Read the model definition and answer for the solid it produces. Units are mm, in the model's axes. A direction names the side the tool comes from. Give positions to 0.01 mm unless a question says otherwise; leave off trailing zeros. Write each loop counter-clockwise with the first axis right and the second up, starting at its lowest first coordinate (ties: lowest second). Pieces come first, ordered by that corner, then holes. Notation, with made-up numbers: M 9.25,49 L 58.25,49 A20 ccw 58.25,63 Z; hole C 49.5,-13.75 d7. An arc over 180 degrees is marked long. Write each question's results on one line, items separated by ' | '. Start each with the question number.
```python
from build123d import *
from build123d.topology import SkipClean

# Parameters (mm, degrees)
SKETCH_1_W               = 49.5
SKETCH_1_H               = 24.5
EXTRUDE_1_DEPTH          = 36
SKETCH_2_R               = 2.5
CUT_EXTRUDE_1_DEPTH      = 3
SKETCH_3_W               = 15.2
SKETCH_3_H               = 2.5
CUT_EXTRUDE_2_DEPTH      = 12
FILLET_1_R               = 3
CUT_EXTRUDE_3_DEPTH      = 46.372072908
CUT_EXTRUDE_3_DEPTH_BACK = 46.372072908
SKETCH_5_R               = 1.95
CUT_EXTRUDE_4_DEPTH      = 63.42044953
CUT_EXTRUDE_4_DEPTH_BACK = 3
SKETCH_6_R               = 4
SKETCH_7_W               = 10
SKETCH_7_H               = 9
CUT_EXTRUDE_5_DEPTH      = 7.5
CUT_EXTRUDE_6_DEPTH      = 63.42044953
FILLET_2_R               = 4
SKETCH_9_W               = 15
SKETCH_9_H               = 30
CUT_EXTRUDE_7_DEPTH      = 15
SKETCH_11_W              = 14.5
SKETCH_11_H              = 1.9
CUT_EXTRUDE_8_DEPTH      = 2


with BuildPart() as part:
    # Эскиз1 → Бобышка-Вытянуть1 (new body)
    with BuildSketch(Plane(origin=(0, 0, 0), x_dir=(0, 0, -1), z_dir=(1, 0, 0))):
        Rectangle(SKETCH_1_W, SKETCH_1_H)
    extrude(amount=EXTRUDE_1_DEPTH)

    # Эскиз2 → Вырез-Вытянуть1 (cut)
    with BuildSketch(Plane.ZY):
        with Locations((-20, -7.25)):
            Circle(SKETCH_2_R)
        with Locations((20, -7.25)):
            Circle(SKETCH_2_R)
    extrude(amount=-CUT_EXTRUDE_1_DEPTH, mode=Mode.SUBTRACT)

    # Эскиз3 → Вырез-Вытянуть2 (cut)
    with BuildSketch(Plane.ZY):
        with Locations((0, 4.75)):
            Rectangle(SKETCH_3_W, SKETCH_3_H)
        with Locations((0, 8.75)):
            Rectangle(SKETCH_3_W, SKETCH_3_H)
    extrude(amount=-CUT_EXTRUDE_2_DEPTH, mode=Mode.SUBTRACT)

    # Скругление1
    fillet_1_edges = [part.edges().sort_by_distance(p)[0] for p in [
        (18, 12.25, -24.75),
        (18, -12.25, -24.75),
        (18, -12.25, 24.75),
        (18, 12.25, 24.75),
    ]]
    fillet(fillet_1_edges, radius=FILLET_1_R)

    # Эскиз5 → Вырез-Вытянуть3 (cut, two sides: drawn at the far end of the back side and taken through both)
    with BuildSketch(Plane.XY.offset(-CUT_EXTRUDE_3_DEPTH_BACK)):
        with Locations(Location((29, -8.25, 0), (0, 0, 329.148114014))):
            Circle(SKETCH_5_R)
    extrude(amount=CUT_EXTRUDE_3_DEPTH + CUT_EXTRUDE_3_DEPTH_BACK, mode=Mode.SUBTRACT)

    # Эскиз6 → Вырез-Вытянуть4 (cut, two sides: drawn at the far end of the back side and taken through both)
    with BuildSketch(Plane(origin=(0, 0, -24.75), x_dir=(-1, 0, 0), z_dir=(0, 0, -1)).offset(-CUT_EXTRUDE_4_DEPTH_BACK)):
        with Locations((-29, -8.25)):
            Circle(SKETCH_6_R)
    extrude(amount=CUT_EXTRUDE_4_DEPTH + CUT_EXTRUDE_4_DEPTH_BACK, mode=Mode.SUBTRACT)

    # Эскиз7 → Вырез-Вытянуть5 (cut, symmetric)
    with SkipClean():  # the faces are left unmerged after this step: merging them gives an invalid solid
        with BuildSketch(Plane.XY):
            with Locations((29, -7.75)):
                Rectangle(SKETCH_7_W, SKETCH_7_H)
        extrude(amount=CUT_EXTRUDE_5_DEPTH, both=True, mode=Mode.SUBTRACT)

    # Эскиз8 → Вырез-Вытянуть6 (cut, through all)
    with SkipClean():  # the faces are left unmerged after this step: merging them gives an invalid solid
        with BuildSketch(Plane(origin=(0, 0, -24.75), x_dir=(-1, 0, 0), z_dir=(0, 0, -1))):
            Polygon((-11, 12.25), (-36, -2.25), (-36, 12.25), align=None)
        extrude(amount=-CUT_EXTRUDE_6_DEPTH, mode=Mode.SUBTRACT)

    # Скругление2
    fillet_2_edges = [part.edges().sort_by_distance(p)[0] for p in [
        (36, -2.25, 0),
    ]]
    fillet(fillet_2_edges, radius=FILLET_2_R)

    # Эскиз9 → Вырез-Вытянуть7 (cut)
    with BuildSketch(Plane.XZ.offset(-12.25)):
        with Locations((20.5, 0)):
            Rectangle(SKETCH_9_W, SKETCH_9_H)
    extrude(amount=CUT_EXTRUDE_7_DEPTH, mode=Mode.SUBTRACT)

    # Эскиз11 → Вырез-Вытянуть8 (cut)
    with BuildSketch(Plane.ZY.offset(-12)):
        with Locations((0, 8.75)):
            Rectangle(SKETCH_11_W, SKETCH_11_H)
        with Locations((0, 4.75)):
            Rectangle(SKETCH_11_W, SKETCH_11_H)
    extrude(amount=-CUT_EXTRUDE_8_DEPTH, mode=Mode.SUBTRACT)


solid = part.part
```
Item 1: Section A-A, the plane z = 4 is taken. Give the number of separate pieces and of enclosed holes in the cut face, then the cut area to 3 significant figures.
Item 2: Section C-C, the plane x = 10 is taken. Determine the outline of the cut face in (y, z).
Item 3: Given P1, Ø1, axis at y = 8.5, z = -3, coming from the +X side; P2, Ø3, axis at x = 27.5, z = -2.5, coming from the -Y side; P3, Ø0.8, axis at x = 12.5, z = 1.5, coming from the +Y side; P4, Ø10, axis at x = 13.5, z = 10, coming from the +Y side, each flat-ended and moving along its own axis, determine where each tip first touches the part or whether it passes through.
Item 4: Straight lines are drawn through the part: line 1 (X direction, y = -8.25, z = -23.1); line 2 (Z direction, x = 14, y = 0.25); line 3 (X direction, y = -5.25, z = -4.5). For each, find the intervals that lie inside material, in ascending order.
Item 5: Determine the mould class of faces 4 (the flat face through (34, -8, 0)), 5 (the flat face through (14, 0, 24.75)), 6 (the cylindrical face through (35.45, -2.53, 0.35)) for opening direction X: +X half, -X half, draft (parallel to the pull), parting line (faces both ways), or undercut.
Item 6: Section D-D, the plane x = 19 is taken. Determine the outline of the cut face in (y, z).
Item 7: For faces 1 (the flat face through (3, -7, 20)), 2 (the cylindrical face through (29.521, -4.284, -23.229)), 3 (the flat face through (12.5, 4.7, -7.25)), determine the directions among +Z, -Z, +X, -X, +Y, -Y from which every point of the face is accessible in a straight line to the end or side of a thin tool.
Item 8: Section B-B, the plane y = 4.5 is taken. Determine the outline of the cut face in (x, z).
Worked out:
1) separate pieces: 3 | enclosed holes: 0 | area: 404 mm²
2) outline: M -12.25,-21.75 A3 ccw -9.25,-24.75 L 9.25,-24.75 A3 ccw 12.25,-21.75 L 12.25,21.75 A3 ccw 9.25,24.75 L -9.25,24.75 A3 ccw -12.25,21.75 Z; hole M 3.5,-7.6 L 6,-7.6 L 6,7.6 L 3.5,7.6 Z; hole M 7.5,-7.6 L 10,-7.6 L 10,7.6 L 7.5,7.6 Z
3) P1: passes through | P2: stops at y = -3.25 | P3: stops at y = 11.61 | P4: stops at y = 12.25
4) line 1: x = 0 to 25, 33 to 36 | line 2: z = -24.75 to -15, 15 to 24.75 | line 3: x = 0 to 24, 34 to 36
5) face 4: undercut | face 5: draft | face 6: +X half
6) outline: M -12.25,-21.75 A3 ccw -9.25,-24.75 L 7.61,-24.75 L 7.61,-15 L -2.75,-15 L -2.75,15 L 7.61,15 L 7.61,24.75 L -9.25,24.75 A3 ccw -12.25,21.75 Z
7) face 1: -X | face 2: -Z | face 3: +X, -X
8) outline: M 0,-24.75 L 24.36,-24.75 L 24.36,-15 L 13,-15 L 13,-7.25 L 12,-7.25 L 12,-7.6 L 0,-7.6 Z; M 0,7.6 L 12,7.6 L 12,7.25 L 13,7.25 L 13,15 L 24.36,15 L 24.36,24.75 L 0,24.75 Z
